```python
from build123d import *
from build123d.topology import SkipClean

# Parameters (mm, degrees)
SALIENTE_EXTRUIR1_DEPTH      = 2
SALIENTE_EXTRUIR1_DEPTH_BACK = 2
CROQUIS2_R                   = 26.5
SALIENTE_EXTRUIR2_DEPTH      = 22
SALIENTE_EXTRUIR2_DEPTH_BACK = 22
CROQUIS3_R                   = 11
CROQUIS5_W                   = 5
CROQUIS5_H                   = 10.605029608
SALIENTE_EXTRUIR3_DEPTH      = 14
SALIENTE_EXTRUIR5_DEPTH      = 14
CROQUIS7_W                   = 24.5
CROQUIS7_H                   = 19
SALIENTE_EXTRUIR12_DEPTH     = 21
CROQUIS8_R                   = 2
CORTAR_EXTRUIR1_DEPTH        = 37
CROQUIS10_W                  = 24.5
CROQUIS10_H                  = 19
CORTAR_EXTRUIR2_DEPTH        = 19
MATRIZC2_COUNT               = 3
CORTAR_EXTRUIR3_START        = -19
CORTAR_EXTRUIR3_DEPTH        = 19
CORTAR_EXTRUIR5_DEPTH        = 33
CORTAR_EXTRUIR5_DEPTH_BACK   = 33
CROQUIS15_W                  = 59.132564764
CROQUIS15_H                  = 24.236023023
CROQUIS16_R                  = 0.5
CORTAR_EXTRUIR6_DEPTH        = 10
CROQUIS17_W                  = 2.150315422
CROQUIS17_H                  = 1
CROQUIS17_W_2                = 1
CROQUIS17_H_2                = 1.647197796
CORTAR_EXTRUIR8_DEPTH        = 0.1


with BuildPart() as part:
    # Croquis2 → Saliente-Extruir1 (new, two sides: drawn at the far end of the back side and taken through both)
    with BuildSketch(Plane(origin=(0, 0, 0), x_dir=(1, 0, 0), z_dir=(0, 1, 0)).offset(-SALIENTE_EXTRUIR1_DEPTH_BACK)):
        with Locations(Location((0, 0, 0), (0, 0, 270))):
            Circle(CROQUIS2_R)
    extrude(amount=SALIENTE_EXTRUIR1_DEPTH + SALIENTE_EXTRUIR1_DEPTH_BACK)

    # Croquis3 → Saliente-Extruir2 (add, two sides: drawn at the far end of the back side and taken through both)
    with BuildSketch(Plane(origin=(0, 0, 0), x_dir=(1, 0, 0), z_dir=(0, 1, 0)).offset(-SALIENTE_EXTRUIR2_DEPTH_BACK)):
        with Locations(Location((0, 0, 0), (0, 0, 270))):
            Circle(CROQUIS3_R)
        Polygon((0, 6.639528096), (-5.75, 3.319764048), (-5.75, -3.319764048), (0, -6.639528096), (5.75, -3.319764048), (5.75, 3.319764048), align=None, mode=Mode.SUBTRACT)
    extrude(amount=SALIENTE_EXTRUIR2_DEPTH + SALIENTE_EXTRUIR2_DEPTH_BACK)

    # Croquis5 → Saliente-Extruir3 (add)
    with BuildSketch(Plane(origin=(0, 0, 0), x_dir=(1, 0, 0), z_dir=(0, 1, 0))):
        with Locations((0, 13.697485196)):
            Rectangle(CROQUIS5_W, CROQUIS5_H)
        Polygon((8.520257623, -2.032421687), (17.704482672, -7.334936491), (15.204482672, -11.665063509), (6.020257623, -6.362548705), align=None)
        Polygon((-6.020257623, -6.362548705), (-15.204482672, -11.665063509), (-17.704482672, -7.334936491), (-8.520257623, -2.032421687), align=None)
    extrude(amount=SALIENTE_EXTRUIR3_DEPTH)

    # Croquis6 → Saliente-Extruir5 (add)
    with BuildSketch(Plane(origin=(0, 0, 0), x_dir=(1, 0, 0), z_dir=(0, 1, 0))):
        with BuildLine():
            Line((-12.25, -11), (-12.25, -24))
            Line((-12.25, -24), (-13, -24))
            ThreePointArc((-13, -24), (-15.828427125, -22.828427125), (-17, -20))
            Line((-17, -20), (-17, -9))
            Line((-17, -9), (-12.25, -9))
            Line((-12.25, -9), (-12.25, -11))
        make_face()
        with BuildLine():
            Line((12.25, -11), (12.25, -24))
            Line((12.25, -24), (13, -24))
            ThreePointArc((13, -24), (15.828427125, -22.828427125), (17, -20))
            Line((17, -20), (17, -9))
            Line((17, -9), (12.25, -9))
            Line((12.25, -9), (12.25, -11))
        make_face()
        with BuildLine():
            Line((-1.669228634, 15.108811196), (0.705771366, 19.222431864))
            Line((0.705771366, 19.222431864), (-8.820508076, 24.722431864))
            ThreePointArc((-8.820508076, 24.722431864), (-11.855784256, 25.122033554), (-14.284609691, 23.258330249))
            Line((-14.284609691, 23.258330249), (-14.659609691, 22.608811196))
            Line((-14.659609691, 22.608811196), (-3.401279442, 16.108811196))
            Line((-3.401279442, 16.108811196), (-1.669228634, 15.108811196))
        make_face()
        with BuildLine():
            Line((-15.651279442, -5.108811196), (-26.909609691, 1.391188804))
            Line((-26.909609691, 1.391188804), (-27.284609691, 0.741669751))
            ThreePointArc((-27.284609691, 0.741669751), (-27.684211381, -2.29360643), (-25.820508076, -4.722431864))
            Line((-25.820508076, -4.722431864), (-16.294228634, -10.222431864))
            Line((-16.294228634, -10.222431864), (-13.919228634, -6.108811196))
            Line((-13.919228634, -6.108811196), (-15.651279442, -5.108811196))
        make_face()
        with BuildLine():
            Line((13.919228634, -6.108811196), (16.294228634, -10.222431864))
            Line((16.294228634, -10.222431864), (25.820508076, -4.722431864))
            ThreePointArc((25.820508076, -4.722431864), (27.684211381, -2.29360643), (27.284609691, 0.741669751))
            Line((27.284609691, 0.741669751), (26.909609691, 1.391188804))
            Line((26.909609691, 1.391188804), (15.651279442, -5.108811196))
            Line((15.651279442, -5.108811196), (13.919228634, -6.108811196))
        make_face()
        with BuildLine():
            Line((3.401279442, 16.108811196), (14.659609691, 22.608811196))
            Line((14.659609691, 22.608811196), (14.284609691, 23.258330249))
            ThreePointArc((14.284609691, 23.258330249), (11.855784256, 25.122033554), (8.820508076, 24.722431864))
            Line((8.820508076, 24.722431864), (-0.705771366, 19.222431864))
            Line((-0.705771366, 19.222431864), (1.669228634, 15.108811196))
            Line((1.669228634, 15.108811196), (3.401279442, 16.108811196))
        make_face()
    extrude(amount=SALIENTE_EXTRUIR5_DEPTH)

    # Croquis7 → Saliente-Extruir12 (add)
    with BuildSketch(Plane(origin=(0, 0, 0), x_dir=(1, 0, 0), z_dir=(0, 1, 0))):
        with Locations((0, -20.6)):
            Rectangle(CROQUIS7_W, CROQUIS7_H)
    extrude(amount=SALIENTE_EXTRUIR12_DEPTH)

    # Croquis8 → Cortar-Extruir1 (cut, symmetric)
    with BuildSketch(Plane(origin=(12.25, 0, 0), x_dir=(0, 0, -1), z_dir=(1, 0, 0))):
        with Locations(Location((-20.6, 11.5, 0), (0, 0, 72.542396876))):
            Circle(CROQUIS8_R)
    cortar_extruir1 = extrude(amount=CORTAR_EXTRUIR1_DEPTH, both=True, mode=Mode.SUBTRACT)

    # Croquis10 → Cortar-Extruir2 (cut)
    with BuildSketch(Plane(origin=(0, 21, 0), x_dir=(1, 0, 0), z_dir=(0, 1, 0))):
        with Locations((0, -20.6)):
            Rectangle(CROQUIS10_W, CROQUIS10_H)
    extrude(amount=-CORTAR_EXTRUIR2_DEPTH, mode=Mode.SUBTRACT)

    # MatrizC2: Cortar-Extruir1 ×3 about axis
    matrizc2_axis = Axis((0, -24.2, 0), (0, 1, 0))
    for i in range(1, MATRIZC2_COUNT):
        add(cortar_extruir1.rotate(matrizc2_axis, i * 360 / MATRIZC2_COUNT), mode=Mode.SUBTRACT)

    # Croquis14 → Cortar-Extruir3 (cut)
    with SkipClean():  # the faces are left unmerged after this step: merging them gives an invalid solid
        with BuildSketch(Plane(origin=(0, 2, 0), x_dir=(1, 0, 0), z_dir=(0, 1, 0)).offset(CORTAR_EXTRUIR3_START)):
            with BuildLine():
                Line((-12.25, -24), (-12.25, -30.1))
                Line((-12.25, -30.1), (12.25, -30.1))
                Line((12.25, -30.1), (12.25, -24))
                Line((12.25, -24), (12.25, -23.498670175))
                ThreePointArc((12.25, -23.498670175), (0, -26.5), (-12.25, -23.498670175))
                Line((-12.25, -23.498670175), (-12.25, -24))
            make_face()
        extrude(amount=CORTAR_EXTRUIR3_DEPTH, mode=Mode.SUBTRACT)

    # Croquis15 → Cortar-Extruir5 (cut, two sides: drawn at the far end of the back side and taken through both)
    with BuildSketch(Plane.XY.offset(-CORTAR_EXTRUIR5_DEPTH_BACK)):
        with Locations((-0.66628242, -12.118011512)):
            Rectangle(CROQUIS15_W, CROQUIS15_H)
    extrude(amount=CORTAR_EXTRUIR5_DEPTH + CORTAR_EXTRUIR5_DEPTH_BACK, mode=Mode.SUBTRACT)

    # Croquis16 → Cortar-Extruir6 (cut)
    with BuildSketch(Plane(origin=(0, 2, 0), x_dir=(1, 0, 0), z_dir=(0, 1, 0))):
        with Locations(Location((0, 0, 0), (0, 0, 270))):
            Circle(CROQUIS16_R)
    extrude(amount=-CORTAR_EXTRUIR6_DEPTH, mode=Mode.SUBTRACT)

    # Croquis17 → Cortar-Extruir8 (cut)
    with BuildSketch(Plane.XZ):
        Rectangle(CROQUIS17_W, CROQUIS17_H)
        Rectangle(CROQUIS17_W_2, CROQUIS17_H_2)
    extrude(amount=-CORTAR_EXTRUIR8_DEPTH, mode=Mode.SUBTRACT)


solid = part.part
```
Could you check a few things on this model? Use its own coordinates, in mm. A direction names the side the tool comes from. Round coordinates to 2 decimals unless told otherwise and drop trailing zeros. Loops run counter-clockwise (first coordinate to the right, second up) from the corner with the lowest first, then second, coordinate; pieces in that order, holes last. Notation, with made-up numbers: M -21,-9.75 L 26,-9.75 A38 ccw 26,28.25 Z; hole C 63,-32.75 d4. An arc over 180 degrees is marked long. Write item = value, one per line.
1. I want a section at C-C, the plane x = 21.5. Write out the boundary of the cut face in (y, z).
Results below:
outline = M 0,-15.49 L 2,-15.49 L 2,1.73 L 14,1.73 L 14,7.22 L 2,7.22 L 2,15.49 L 0,15.49 Z
2. Which directions (+Z, -Z, +X, -X, +Y, -Y) give clear straight access to the entire face, cutting with the end or side of a thin tool? Please do faces 1 (the face through (-2.915, 11.86, 4.956)), 2 (the face through (0.1, 1, -26.5)), 3 (the face through (-23.015, 0.986, 13.137)), 4 (the face through (-20, 2, 12)), 5 (the face through (21.349, 7.916, 7.304)).
Results below:
face_1 = +Y
face_2 = -Z, +Y, -Y
face_3 = +Z, -X, +Y, -Y
face_4 = +Z, -X, +Y
face_5 = +Z, +X, +Y
3. Thinking about a two-plate mould opening in Z: for faces 6 (the face through (-21.472, 7.916, 7.233)), 7 (the face through (8.8, 11.8, -22)), 8 (the face through (-16, 14, 10)), which applies, +Z half, -Z half, draft (parallel to the pull), parting line (faces both ways), or undercut?
Results below:
face_6 = +Z half
face_7 = undercut
face_8 = draft
4. Will these pins go through, and if not, where does the flat tip stop? P1, Ø3.5, axis at x = 0, z = 2, coming from the +Y side; P2, Ø4.5, axis at y = 11.5, z = 20.6, coming from the -X side; P3, Ø1, axis at x = -12.5, y = 3, coming from the +Z side.
Results below:
P1 = 2
P2 = -17
P3 = 24
5. I want a section at A-A, the plane y = 15.25. Write out the boundary of the cut face in (x, z).
Results below:
outline = C 0,0 d22; hole M -5.75,-3.32 L 0,-6.64 L 5.75,-3.32 L 5.75,3.32 L 0,6.64 L -5.75,3.32 Z
6. I want a section at B-B, the plane z = -14. Write out the boundary of the cut face in (x, y), and give its area (3 significant figures).
Results below:
outline = M -22.5,0 L 22.5,0 L 22.5,2 L 2.5,2 L 2.5,14 L -2.5,14 L -2.5,2 L -22.5,2 Z
area = 150 mm²
7. I need wall thicknesses on probe 1 along X at (y, z) = (11.5, 17); probe 2 along Y at (x, z) = (-15.9, 20.6); probe 3 along Z at (x, y) = (-5, 4). Which ranges of each line are inside material? Lowest first, please.
Results below:
probe_1 = -17 to -12.25, 12.25 to 17
probe_2 = 0 to 9.5, 13.5 to 14
probe_3 = -22.52 to -17.03, -9.8 to -3.75, 3.75 to 9.8
8. I want a section at D-D, the plane y = 11.5. Count the separate pieces of the cut face and the enclosed holes in it, and give its area (3 significant figures).
Results below:
separate_pieces = 7
enclosed_holes = 1
area = 639 mm²
